```python
from build123d import *

# Parameters (mm, degrees)
SKETCH_1_R          = 1.5
EXTRUDE_1_DEPTH     = 23
SKETCH_1_3_R        = 1.5
EXTRUDE_2_DEPTH     = 19.5
SKETCH_1_6_R        = 11
SKETCH_1_6_R_2      = 2.5
EXTRUDE_4_DEPTH     = 25
SKETCH_2_R          = 4.5
CUT_EXTRUDE_1_DEPTH = 3


with BuildPart() as part:
    # Sketch 1 → Extrude 1 (new body)
    with BuildSketch(Plane.XY):
        Polygon((-21, -17), (-17, -21), (17, -21), (21, -17), (21, 17), (17, 21), (-17, 21), (-21, 17), align=None)
        with Locations((-15.5, -15.5)):
            Circle(SKETCH_1_R, mode=Mode.SUBTRACT)
        with Locations((15.5, -15.5)):
            Circle(SKETCH_1_R, mode=Mode.SUBTRACT)
        with Locations((-15.5, 15.5)):
            Circle(SKETCH_1_R, mode=Mode.SUBTRACT)
        with Locations((15.5, 15.5)):
            Circle(SKETCH_1_R, mode=Mode.SUBTRACT)
    extrude(amount=EXTRUDE_1_DEPTH)

    # Sketch 1_3 → Extrude 2 (add)
    with BuildSketch(Plane.XY):
        with Locations((-15.5, 15.5)):
            Circle(SKETCH_1_3_R)
        with Locations((15.5, 15.5)):
            Circle(SKETCH_1_3_R)
        with Locations(Location((-15.5, -15.5, 0), (0, 0, 180))):
            Circle(SKETCH_1_3_R)
        with Locations(Location((15.5, -15.5, 0), (0, 0, 180))):
            Circle(SKETCH_1_3_R)
    extrude(amount=EXTRUDE_2_DEPTH)

    # Sketch 1_6 → Extrude 4 (add)
    # profile 1 of 5: a face of its own
    with BuildSketch(Plane.XY):
        Circle(SKETCH_1_6_R)
        Circle(SKETCH_1_6_R_2, mode=Mode.SUBTRACT)
    # profile 2 of 5: a face of its own
    with BuildSketch(Plane.XY):
        with BuildLine():
            ThreePointArc((1.5, 2), (0, 2.5), (-1.5, 2))
            Line((-1.5, 2), (1.5, 2))
        make_face()
    # profile 3 of 5: a face of its own
    with BuildSketch(Plane.XY):
        with BuildLine():
            Line((1.5, 2), (-1.5, 2))
            ThreePointArc((-1.5, 2), (-1.118033989, -2.236067977), (2.5, 0))
            ThreePointArc((2.5, 0), (2.236067977, 1.118033989), (1.5, 2))
        make_face()
    # profile 4 of 5: a face of its own
    with BuildSketch(Plane.XY):
        with BuildLine():
            ThreePointArc((1.5, 2), (0, 2.5), (-1.5, 2))
            Line((-1.5, 2), (1.5, 2))
        make_face()
    # profile 5 of 5: a face of its own
    with BuildSketch(Plane.XY):
        with BuildLine():
            Line((1.5, 2), (-1.5, 2))
            ThreePointArc((-1.5, 2), (-1.118033989, -2.236067977), (2.5, 0))
            ThreePointArc((2.5, 0), (2.236067977, 1.118033989), (1.5, 2))
        make_face()
    extrude(amount=EXTRUDE_4_DEPTH)

    # Sketch 2 → Cut-Extrude 1 (cut)
    with BuildSketch(Plane.XY.offset(25)):
        Circle(SKETCH_2_R)
    extrude(amount=-CUT_EXTRUDE_1_DEPTH, mode=Mode.SUBTRACT)


solid = part.part
```
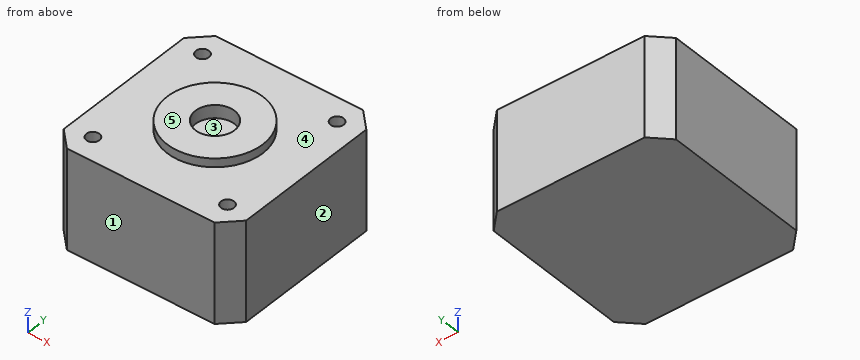
Check sheet for the modelled part. Datum: model origin and axes. Units: mm. Face numbers are marked on the shaded views. A direction names the side the tool comes from. Round coordinates to 2 decimals unless told otherwise and drop trailing zeros. Loops run counter-clockwise (first coordinate to the right, second up) from the corner with the lowest first, then second, coordinate; pieces in that order, holes last. Notation, with made-up numbers: (46, 45) - (101, 45) arc R21 cw to (101, 81) - close; hole circle Ø4 at (8.25, 60.5). An arc over 180 degrees is marked (long way). Answer as a JSON object with one key per item and string values. Group by question number.
Q1. Scan lines: line 1 along X through (y, z) = (-15.5, 21); line 2 along Z through (x, y) = (2.5, 0). Record each from-to range of solid material in increasing order. Write a range as [from, to].
Q2. Sectioned sample at C-C, the plane y = -1. Enter the section's corners in (x, z), plus the area to 3 significant figures.
Q3. Sectioned sample at A-A, the plane x = 0. Enter the section's corners in (y, z).
Q4. Gauge pin test, flat ends, axial feed: P1, Ø1.5, axis at x = -15, y = 15.5, coming from the +Z side; P2, Ø10, axis at x = -15, y = -11, coming from the +Z side. Record the tip position at first contact, or that the pin passes through.
Q5. Set-up check for the marked faces 4 and 5: record each of +Z, -Z, +X, -X, +Y, -Y from which the full face is reachable in a straight line by a thin tool's end or side.
Q6. Sectioned sample at D-D, the plane x = 8.5. Enter the section's corners in (y, z), plus the area to 3 significant figures.
Q7. Sectioned sample at B-B, the plane z = 15. Enter the section's corners in (x, y).
Q8. Mould release check, pull along Y, two halves, no side actions. Record for the marked faces 1, 2 and 3: released by +Y, released by -Y, zero draft, split by the parting line, or undercut.
Solution:
{
 "1": {"line 1": "x = [-21, -17], [-14, 14], [17, 21]", "line 2": "z = [0, 22]"},
 "2": {"outline": "(-21, 0) - (21, 0) - (21, 23) - (10.95, 23) - (10.95, 25) - (4.39, 25) - (4.39, 22) - (-4.39, 22) - (-4.39, 25) - (-10.95, 25) - (-10.95, 23) - (-21, 23) - close", "area": "983 mm²"},
 "3": {"outline": "(-21, 0) - (21, 0) - (21, 23) - (11, 23) - (11, 25) - (4.5, 25) - (4.5, 22) - (-4.5, 22) - (-4.5, 25) - (-11, 25) - (-11, 23) - (-21, 23) - close"},
 "4": {"P1": "stops at z = 19.5", "P2": "stops at z = 23"},
 "5": {"face 4": "+Z", "face 5": "+Z, +X, -X, +Y, -Y"},
 "6": {"outline": "(-21, 0) - (21, 0) - (21, 23) - (6.98, 23) - (6.98, 25) - (-6.98, 25) - (-6.98, 23) - (-21, 23) - close", "area": "994 mm²"},
 "7": {"outline": "(-21, -17) - (-17, -21) - (17, -21) - (21, -17) - (21, 17) - (17, 21) - (-17, 21) - (-21, 17) - close"},
 "8": {"face 1": "released by -Y", "face 2": "zero draft", "face 3": "undercut"}
}
